```python
from build123d import *

# Parameters (mm, degrees)
F0_W          = 53.6921843886
F0_H          = 53.6921843886
F1_DEPTH      = 46.228
F1_TAPER      = 30
F1_DEPTH_BACK = 46.228
F1_TAPER_BACK = 30


with BuildPart() as f1:
    # F0 (on Top) → F1 (new body, two sides)
    with BuildSketch(Plane.XY) as f1_sk:
        with Locations((-14.9725442752, 12.4619603157)):
            Rectangle(F0_W, F0_H)
    extrude(amount=F1_DEPTH, taper=F1_TAPER)
    extrude(f1_sk.sketch, amount=-F1_DEPTH_BACK, taper=F1_TAPER_BACK)


solid = f1.part
```
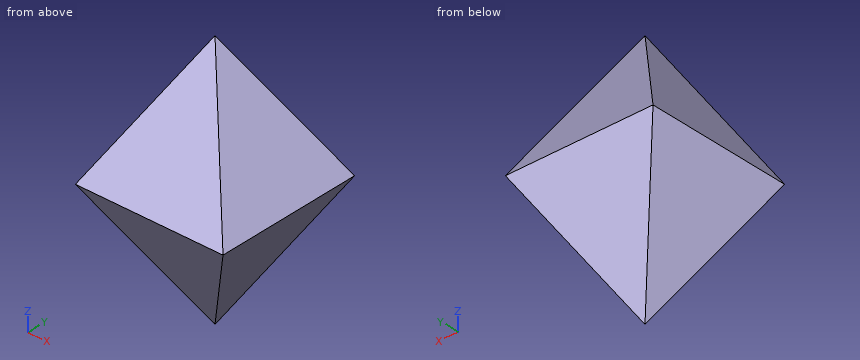
Design review of the part built by this model. Coordinates are the model's own, in mm. Give positions to 0.01 mm unless a question says otherwise; leave off trailing zeros. Order: outer loops, then holes, each group sorted by start corner. A loop starts at its lowest first (then second) coordinate and runs counter-clockwise, first axis right, second up. Notation, with made-up numbers: M 62.5,9 L 113.5,9 A17 cw 113.5,31 Z; hole C 41.5,40.5 d2. An arc over 180 degrees is marked long. One line per question, with ' | ' between items. Start each with the question number.
Q1. We need section B-B (z = 29). Write out the cut boundary in (x, y), plus the area to 3 significant figures.
Q2. We need section A-A (z = 10). Write out the cut boundary in (x, y).
Q3. For L1, parallel to Z at x = -11, y = 17.5; L2, parallel to Z at x = 9, y = 11; L3, parallel to Y at x = -24, z = 21, list the stretches that pass through material, from the lowest coordinate up. Write a range as [from, to].
Q4. For pin 1 Ø4 at (y, z) = (21.5, -29.5) entering from -X; pin 2 Ø3 at (x, y) = (-30, 0) entering from +Z; pin 3 Ø5 at (x, z) = (-13, -12) entering from +Y, all flat-tipped, find the tip position at first contact; note any pin that passes through.
Returned:
1) outline: M -25.08,2.36 L -4.87,2.36 L -4.87,22.56 L -25.08,22.56 Z | area: 408 mm2
2) outline: M -36.05,-8.61 L 6.1,-8.61 L 6.1,33.53 L -36.05,33.53 Z
3) L1: [-37.77, 37.77] | L2: [-4.98, 4.98] | L3: [-2.26, 27.18]
4) pin 1: x = -25.94 | pin 2: z = 23.07 | pin 3: y = 33.82
